Here's how the part is built. I have some questions about the finished solid (model axes, mm). Round coordinates to 2 decimals unless told otherwise and drop trailing zeros. Write each loop counter-clockwise with the first axis right and the second up, starting at its lowest first coordinate (ties: lowest second). Pieces come first, ordered by that corner, then holes. Notation, with made-up numbers: (81, 16.5) -> (90, 16.5) arc R9 cw to (90, 29.5) -> close; hole circle Ø3 at (2, 0.5). An arc over 180 degrees is marked (long way). Answer as CSV lines item,"result".
```python
from build123d import *

# Parameters (mm, degrees)
F0_W     = 38.1
F0_H     = 38.1
F1_DEPTH = 3.048
F2_R     = 15.875
F3_DEPTH = 1.27
F5_DEPTH = 38.101
F7_DEPTH = 38.101


with BuildPart() as f1:
    # F0 (on Top) → F1 (new body)
    with BuildSketch(Plane.XY):
        Rectangle(F0_W, F0_H)
    extrude(amount=F1_DEPTH)

    # F2 (on face) → F3 (cut)
    with BuildSketch(Plane.XY.offset(3.048)):
        Circle(F2_R)
    extrude(amount=-F3_DEPTH, mode=Mode.SUBTRACT)

    # F4 (on face) → F5 (cut, through all)
    with BuildSketch(Plane.XZ.offset(19.05)):
        Polygon((-18.415, 3.048), (-19.05, 3.048), (-19.05, 2.413), align=None)
        Polygon((19.05, 3.048), (18.415, 3.048), (19.05, 2.413), align=None)
    extrude(amount=-F5_DEPTH, mode=Mode.SUBTRACT)

    # F6 (on face) → F7 (cut, through all)
    with BuildSketch(Plane(origin=(-19.05, 0, 0), x_dir=(0, -1, 0), z_dir=(-1, 0, 0))):
        Polygon((-18.415, 3.048), (-19.05, 3.048), (-19.05, 2.413), align=None)
        Polygon((18.415, 3.048), (19.05, 2.413), (19.05, 3.048), align=None)
    extrude(amount=-F7_DEPTH, mode=Mode.SUBTRACT)


solid = f1.part
```
1. Suppose I cut it at A-A on x = 0. Please give me the cut outline in (y, z) (3 decimals), and give its area (3 significant figures).
Numbers:
outline,"(-19.05, 0) -> (19.05, 0) -> (19.05, 2.413) -> (18.415, 3.048) -> (15.875, 3.048) -> (15.875, 1.778) -> (-15.875, 1.778) -> (-15.875, 3.048) -> (-18.415, 3.048) -> (-19.05, 2.413) -> close"
area,"75.4 mm^2"
2. For pin 1 Ø1 at (x, y) = (11, -9) entering from +Z; pin 2 Ø5 at (x, y) = (-9, 1.5) entering from -Z, each with a flat end and sliding along its axis, tell me the tip position at first contact or that it passes through.
Numbers:
pin 1,"stops at z = 1.78"
pin 2,"stops at z = 0"
3. If we mould it in two halves opening along Y, with no side actions, what happens to faces 1 (the face through (0, -19.05, 1)), 2 (the face through (0, 0, 1.778)), 3 (the face through (-19.05, 0, 1)), 4 (the face through (-3.441, -15.497, 2.422))? For each: released by +Y, released by -Y, zero draft, split by the parting line, or undercut.
Numbers:
face 1,"released by -Y"
face 2,"undercut"
face 3,"zero draft"
face 4,"undercut"
4. If I drill on line 1 (Y direction, x = 0, z = 2.1) (3 decimals); line 2 (X direction, y = 1, z = 2.7); line 3 (X direction, y = -6.5, z = 2.05), over which ranges is the centre line in solid material (lowest first)?
Numbers:
line 1,"y = -19.05 to -15.875, 15.875 to 19.05"
line 2,"x = -18.76 to -15.84, 15.84 to 18.76"
line 3,"x = -19.05 to -14.48, 14.48 to 19.05"
